Build history of the part. All positions in model axes, mm. A direction names the side the tool comes from. Give positions to 0.01 mm unless a question says otherwise; leave off trailing zeros. Order: outer loops, then holes, each group sorted by start corner. A loop starts at its lowest first (then second) coordinate and runs counter-clockwise, first axis right, second up. Notation, with made-up numbers: M 41,17 L 71,17 A11 cw 71,26 Z; hole C -4.75,50 d2. An arc over 180 degrees is marked long. Answer as CSV lines item,"result".
from build123d import *

# Parameters (mm, degrees)
F1_DEPTH = 15.875
F2_DEPTH = 6.35


# Not quite as in the source:
# - a length typed as a fraction of an inch, garbled in the dataset ("3 / 203.2 mm" for 3/8 in), is restored


with BuildPart() as f1:
    # F0 (on Top) → F1 (new body)
    with BuildSketch(Plane.XY):
        with BuildLine():
            Line((927.1, 0), (12.7, 0))
            ThreePointArc((12.7, 0), (11.43, -3.81), (8.128, -6.096))
            Line((8.128, -6.096), (927.1, -6.096))
            Line((927.1, -6.096), (927.1, 0))
        make_face()
        with BuildLine():
            Line((927.1, -6.096), (8.128, -6.096))
            ThreePointArc((8.128, -6.096), (1.016, -13.208), (-6.096, -6.096))
            Line((-6.096, -6.096), (-6.096, 139.7))
            Line((-6.096, 139.7), (-76.2, 139.7))
            Line((-76.2, 139.7), (-76.2, -76.2))
            Line((-76.2, -76.2), (927.1, -76.2))
            Line((927.1, -76.2), (927.1, -6.096))
        make_face()
        with BuildLine():
            ThreePointArc((-6.096, -6.096), (1.016, -13.208), (8.128, -6.096))
            ThreePointArc((8.128, -6.096), (2.54, -5.08), (0, 0))
            Line((0, 0), (0, 139.7))
            Line((0, 139.7), (-6.096, 139.7))
            Line((-6.096, 139.7), (-6.096, -6.096))
        make_face()
    extrude(amount=-F1_DEPTH)

    # F0 (on Top) → F2 (join)
    with BuildSketch(Plane.XY):
        with BuildLine():
            Line((927.1, -6.096), (8.128, -6.096))
            ThreePointArc((8.128, -6.096), (1.016, -13.208), (-6.096, -6.096))
            Line((-6.096, -6.096), (-6.096, 139.7))
            Line((-6.096, 139.7), (-76.2, 139.7))
            Line((-76.2, 139.7), (-76.2, -76.2))
            Line((-76.2, -76.2), (927.1, -76.2))
            Line((927.1, -76.2), (927.1, -6.096))
        make_face()
    extrude(amount=F2_DEPTH)


solid = f1.part
Item 1: Probe line 1 along X through (y, z) = (19, 4); line 2 along X through (y, z) = (86, -13). List the from-to ranges inside material, lowest first. Write a range as from..to.
Geometry says:
line 1,"x = -76.2..-6.1"
line 2,"x = -76.2..0"
Item 2: Drop flat-ended pins along their axis: pin 1 (12.5 mm diameter, centred on x = 417, z = -11, fed in from +Y); pin 2 (5 mm diameter, centred on y = 104, z = -8, fed in from +X); pin 3 (6 mm diameter, centred on y = 45.5, z = 3.5, fed in from +X); pin 4 (6.5 mm diameter, centred on x = 622, y = -3.5, fed in from +Z). Give the stop position or say it passes through.
Geometry says:
pin 1,"stops at y = 0"
pin 2,"stops at x = 0"
pin 3,"stops at x = -6.1"
pin 4,"stops at z = 6.35"
Item 3: 3-axis set-ups, long thin cutter, end or side, ignore diameter. For faces 1 (the flat face through (-38, 139.7, -5)), 2 (the flat face through (476, 0, -8)): which of +Z, -Z, +X, -X, +Y, -Y reach the whole face in a straight line?
Geometry says:
face 1,"+Z, -Z, +X, -X, +Y"
face 2,"+Z, -Z, +X, +Y"
Item 4: Band-saw the part on B-B (x = 755). Give the cut face in (y, z) (3 decimals), and give its area (3 significant figures).
Geometry says:
outline,"M -76.2,-15.875 L 0,-15.875 L 0,0 L -6.096,0 L -6.096,6.35 L -76.2,6.35 Z"
area,"1,650 mm2"
Item 5: Band-saw the part on A-A (z = -9.25). Give the cut face in (x, y), and give its area (3 significant figures).
Geometry says:
outline,"M -76.2,-76.2 L 927.1,-76.2 L 927.1,0 L 12.7,0 A6.35 cw 0,0 L 0,139.7 L -76.2,139.7 Z"
area,"87,000 mm2"
